Work out the finished part from the listing and answer in its coordinate system (mm). Face numbers are marked on the shaded views. A direction names the side the tool comes from. Give positions to 0.01 mm unless a question says otherwise; leave off trailing zeros. Loops run counter-clockwise (first coordinate to the right, second up) from the corner with the lowest first, then second, coordinate; pieces in that order, holes last. Notation, with made-up numbers: M -14.5,-13.75 L 34.5,-13.75 A23 cw 34.5,-5.75 Z; hole C 46.25,70 d1. An arc over 180 degrees is marked long. Use a Markdown table: item, result.
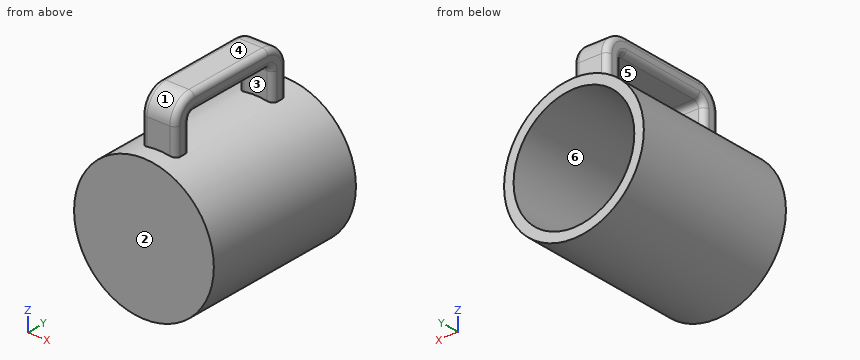
```python
from build123d import *

# Parameters (mm, degrees)
ESBO_O2_W                = 25
ESBO_O2_H                = 60
ESBO_O3_R                = 21.591040813
CORTE_EXTRUS_O1_DEPTH    = 57
RESSALTO_EXTRUS_O1_REACH = 85.869


with BuildPart() as part:
    # Esbo_o2 → Revolu_o1 (revolve)
    with BuildSketch(Plane(origin=(0, 0, 0), x_dir=(0, 0, -1), z_dir=(1, 0, 0)), mode=Mode.PRIVATE) as revolu_o1_sk:
        with Locations((-12.5, 30)):
            Rectangle(ESBO_O2_W, ESBO_O2_H)
    revolve(revolu_o1_sk.sketch.rotate(Axis((0, 0, 0), (0, 1, 0)), 180), axis=Axis((0, 0, 0), (0, 1, 0)))

    # Esbo_o3 → Corte-extrus_o1 (cut)
    with BuildSketch(Plane(origin=(0, 60, 0), x_dir=(1, 0, 0), z_dir=(0, 1, 0))):
        with Locations(Location((0, 0, 0), (0, 0, 270))):
            Circle(ESBO_O3_R)
    extrude(amount=-CORTE_EXTRUS_O1_DEPTH, mode=Mode.SUBTRACT)

    # Esbo_o6 → Ressalto-extrus_o1 (add, up to next)
    with BuildSketch(Plane(origin=(0, 0, 28), x_dir=(-1, 0, 0), z_dir=(0, 0, -1)), mode=Mode.PRIVATE) as ressalto_extrus_o1_sk1:
        with BuildLine():
            Line((4.062337727, 53.13495059), (-4.062337727, 53.13495059))
            ThreePointArc((-4.062337727, 53.13495059), (-5.476551289, 52.549164152), (-6.062337727, 51.13495059))
            Line((-6.062337727, 51.13495059), (-6.062337727, 49.072612863))
            ThreePointArc((-6.062337727, 49.072612863), (-5.476551289, 47.658399301), (-4.062337727, 47.072612863))
            Line((-4.062337727, 47.072612863), (4.062337727, 47.072612863))
            ThreePointArc((4.062337727, 47.072612863), (5.476551289, 47.658399301), (6.062337727, 49.072612863))
            Line((6.062337727, 49.072612863), (6.062337727, 51.13495059))
            ThreePointArc((6.062337727, 51.13495059), (5.476551289, 52.549164152), (4.062337727, 53.13495059))
        make_face()
    ressalto_extrus_o1_tool1 = extrude(ressalto_extrus_o1_sk1.sketch, amount=RESSALTO_EXTRUS_O1_REACH, mode=Mode.PRIVATE) - part.part
    # Esbo_o6 → Ressalto-extrus_o1 (add, up to next)
    with BuildSketch(Plane(origin=(0, 0, 28), x_dir=(-1, 0, 0), z_dir=(0, 0, -1)), mode=Mode.PRIVATE) as ressalto_extrus_o1_sk2:
        with BuildLine():
            Line((6.062337727, 8.119097581), (6.062337727, 10.181435308))
            ThreePointArc((6.062337727, 10.181435308), (5.476551289, 11.59564887), (4.062337727, 12.181435308))
            Line((4.062337727, 12.181435308), (-4.062337727, 12.181435308))
            ThreePointArc((-4.062337727, 12.181435308), (-5.476551289, 11.59564887), (-6.062337727, 10.181435308))
            Line((-6.062337727, 10.181435308), (-6.062337727, 8.119097581))
            ThreePointArc((-6.062337727, 8.119097581), (-5.476551289, 6.704884018), (-4.062337727, 6.119097581))
            Line((-4.062337727, 6.119097581), (4.062337727, 6.119097581))
            ThreePointArc((4.062337727, 6.119097581), (5.476551289, 6.704884018), (6.062337727, 8.119097581))
        make_face()
    ressalto_extrus_o1_tool2 = extrude(ressalto_extrus_o1_sk2.sketch, amount=RESSALTO_EXTRUS_O1_REACH, mode=Mode.PRIVATE) - part.part


with BuildPart() as body_2:
    # Varredura1: sweep along a path in Esbo_o5
    with BuildLine(Plane(origin=(0, 0, 0), x_dir=(0, 0, -1), z_dir=(1, 0, 0))) as varredura1_path:
        Line((-28, 50.103781727), (-34, 50.103781727))
        ThreePointArc((-34, 50.103781727), (-37.535533906, 48.639315633), (-39, 45.103781727))
        Line((-39, 45.103781727), (-39, 14.150266444))
        ThreePointArc((-39, 14.150266444), (-37.535533906, 10.614732538), (-34, 9.150266444))
        Line((-34, 9.150266444), (-28, 9.150266444))
    # Esbo_o4 → Varredura1 (sweep)
    with BuildSketch(Plane.XY.offset(28)):
        with BuildLine():
            Line((-4.062337727, 53.13495059), (4.062337727, 53.13495059))
            ThreePointArc((4.062337727, 53.13495059), (5.476551289, 52.549164152), (6.062337727, 51.13495059))
            Line((6.062337727, 51.13495059), (6.062337727, 49.072612863))
            ThreePointArc((6.062337727, 49.072612863), (5.476551289, 47.658399301), (4.062337727, 47.072612863))
            Line((4.062337727, 47.072612863), (-4.062337727, 47.072612863))
            ThreePointArc((-4.062337727, 47.072612863), (-5.476551289, 47.658399301), (-6.062337727, 49.072612863))
            Line((-6.062337727, 49.072612863), (-6.062337727, 51.13495059))
            ThreePointArc((-6.062337727, 51.13495059), (-5.476551289, 52.549164152), (-4.062337727, 53.13495059))
        make_face()
    sweep(path=varredura1_path.line)


with BuildPart() as part_1:
    add(part.part)

    add(body_2.part)  # Ressalto-extrus_o1 merges body 2
    add(ressalto_extrus_o1_tool1.solids().sort_by_distance((0, 50.103782, 28))[0])
    add(ressalto_extrus_o1_tool2.solids().sort_by_distance((0, 9.150266, 28))[0])


solid = part_1.part
```
(1) A cutting plane is placed at A-A (x = 0). Write down the section's boundary in (y, z).
Entries:
| item | result |
|---|---|
| outline | M 0,-25 L 60,-25 L 60,-21.59 L 3,-21.59 L 3,21.59 L 60,21.59 L 60,25 L 53.13,25 L 53.13,34 A8.03 ccw 45.1,42.03 L 14.15,42.03 A8.03 ccw 6.12,34 L 6.12,25 L 0,25 Z; hole M 12.18,25 L 47.07,25 L 47.07,34 A1.97 ccw 45.1,35.97 L 14.15,35.97 A1.97 ccw 12.18,34 Z |
(2) A cutting plane is placed at B-B (y = 24). Write down the section's boundary in (x, z).
Entries:
| item | result |
|---|---|
| outline | C 0,0 d50; M -6.06,37.97 A2 ccw -4.06,35.97 L 4.06,35.97 A2 ccw 6.06,37.97 L 6.06,40.03 A2 ccw 4.06,42.03 L -4.06,42.03 A2 ccw -6.06,40.03 Z; hole C 0,0 d43.18 |
(3) A cutting plane is placed at C-C (z = 0). Write down the section's boundary in (x, y).
Entries:
| item | result |
|---|---|
| outline | M -25,0 L 25,0 L 25,60 L 21.59,60 L 21.59,3 L -21.59,3 L -21.59,60 L -25,60 Z |
(4) A cutting plane is placed at D-D (y = 54). Write down the section's boundary in (x, z).
Entries:
| item | result |
|---|---|
| outline | C 0,0 d50; hole C 0,0 d43.18 |
(5) Consider probe 1 along X at (y, z) = (27, 0); probe 2 along Z at (x, y) = (2, 21); probe 3 along Y at (x, z) = (-9, 8.5). Determine where each line is inside the solid, lowest interval first. Write a range as [from, to].
Entries:
| item | result |
|---|---|
| probe 1 | x = [-25, -21.59], [21.59, 25] |
| probe 2 | z = [-24.92, -21.5], [21.5, 24.92], [35.97, 42.03] |
| probe 3 | y = [0, 3] |
(6) Which of the six approach directions +Z, -Z, +X, -X, +Y, -Y give full straight-line access (tool end or side, diameter ignored) to the marked faces 4, 5 and 6?
Entries:
| item | result |
|---|---|
| face 4 | +Z, +X, -X, +Y, -Y |
| face 5 | +X, -X |
| face 6 | +Y |
(7) Given P1, Ø5, axis at y = 31, z = 22, coming from the -X side; P2, Ø6, axis at x = -9.5, z = 30, coming from the +Y side; P3, Ø1.5, axis at y = 37.5, z = 2.5, coming from the -X side; P4, Ø10, axis at x = 3.5, y = 9.5, coming from the +Z side, each flat-ended and moving along its own axis, determine where each tip first touches the part or whether it passes through.
Entries:
| item | result |
|---|---|
| P1 | stops at x = -15.64 |
| P2 | passes through |
| P3 | stops at x = -24.94 |
| P4 | stops at z = 42.03 |
(8) The mould has two halves that part along Z. Classify the marked faces 1, 2 and 3: released by +Z, released by -Z, zero draft, split by the parting line, or undercut.
Entries:
| item | result |
|---|---|
| face 1 | released by +Z |
| face 2 | zero draft |
| face 3 | undercut |
